```python
from build123d import *

# Parameters (mm, degrees)
BOSS_EXTRUDE1_DEPTH = 59
FILLET1_R           = 1.5
SKETCH2_W           = 8.5
SKETCH2_H           = 4
CUT_EXTRUDE1_DEPTH  = 145.392693721
LPATTERN1_COUNT     = 15
LPATTERN1_PITCH     = 4.8
SKETCH3_W           = 104
SKETCH3_H           = 71.9
BOSS_EXTRUDE2_DEPTH = 22.5
SKETCH4_W           = 35
SKETCH4_H           = 3.5
CUT_EXTRUDE2_DEPTH  = 1
CUT_EXTRUDE3_REACH  = 104.011
SKETCH8_W           = 11.8
SKETCH8_H           = 90
CUT_EXTRUDE4_DEPTH  = 1
SKETCH9_W           = 9
SKETCH9_H           = 30.5
SKETCH9_H_2         = 31.5
BOSS_EXTRUDE4_DEPTH = 2.8
SKETCH10_W          = 9.9
SKETCH10_H          = 21
BOSS_EXTRUDE5_DEPTH = 1
SKETCH11_R          = 1.5
BOSS_EXTRUDE6_DEPTH = 1
FILLET2_R           = 1


# Read off the part's stored shape, not the designer's step: Dome1, Dome2
with BuildPart() as part:
    # Sketch1 → Boss-Extrude1 (new, symmetric)
    with BuildSketch(Plane.XY):
        Polygon((0, 0), (35, 0), (35, 75.5), (23.5, 75.5), (23.5, 3.5), (0, 3.5), align=None)
    extrude(amount=BOSS_EXTRUDE1_DEPTH, both=True)

    # Fillet1
    fillet1_edges = [part.edges().sort_by_distance(p)[0] for p in [
        (35, 37.75, 59),
        (0, 1.75, 59),
        (35, 37.75, -59),
        (0, 1.75, -59),
    ]]
    fillet(fillet1_edges, radius=FILLET1_R)

    # Sketch2 → Cut-Extrude1 (cut, through all)
    with BuildSketch(Plane.XY.offset(59)):
        with Locations((30.75, 5.5)):
            Rectangle(SKETCH2_W, SKETCH2_H)
    cut_extrude1 = extrude(amount=-CUT_EXTRUDE1_DEPTH, mode=Mode.SUBTRACT)

    # LPattern1: Cut-Extrude1 ×15
    with Locations(*[(0, i * LPATTERN1_PITCH, 0) for i in range(1, LPATTERN1_COUNT)]):
        add(cut_extrude1, mode=Mode.SUBTRACT)

    # Sketch3 → Boss-Extrude2 (add)
    with BuildSketch(Plane.ZY.offset(-23.5)):
        with Locations((0, 39.45)):
            Rectangle(SKETCH3_W, SKETCH3_H)
    extrude(amount=BOSS_EXTRUDE2_DEPTH)

    # Sketch4 → Cut-Extrude2 (cut)
    with BuildSketch(Plane.ZY):
        with Locations((0, 1.75)):
            Rectangle(SKETCH4_W, SKETCH4_H)
    extrude(amount=-CUT_EXTRUDE2_DEPTH, mode=Mode.SUBTRACT)

    # Sketch5 → Cut-Extrude3 (cut, up to next)
    with BuildSketch(Plane.XZ, mode=Mode.PRIVATE) as cut_extrude3_sk1:
        with BuildLine():
            Line((12.75, 59), (12.75, 56))
            ThreePointArc((12.75, 56), (10.5, 53.75), (8.25, 56))
            Line((8.25, 56), (8.25, 59))
            ThreePointArc((8.25, 59), (10.5, 61.25), (12.75, 59))
        make_face()
    cut_extrude3_tool1 = extrude(cut_extrude3_sk1.sketch, amount=-CUT_EXTRUDE3_REACH, mode=Mode.PRIVATE) & part.part
    # Sketch5 → Cut-Extrude3 (cut, up to next)
    with BuildSketch(Plane.XZ, mode=Mode.PRIVATE) as cut_extrude3_sk2:
        with BuildLine():
            Line((12.75, -59), (12.75, -56))
            ThreePointArc((12.75, -56), (10.5, -53.75), (8.25, -56))
            Line((8.25, -56), (8.25, -59))
            ThreePointArc((8.25, -59), (10.5, -61.25), (12.75, -59))
        make_face()
    cut_extrude3_tool2 = extrude(cut_extrude3_sk2.sketch, amount=-CUT_EXTRUDE3_REACH, mode=Mode.PRIVATE) & part.part
    add(cut_extrude3_tool1.solids().sort_by_distance((10.5, 0, 57.5))[0], mode=Mode.SUBTRACT)
    add(cut_extrude3_tool2.solids().sort_by_distance((10.5, 0, -57.5))[0], mode=Mode.SUBTRACT)

    # Sketch8 → Cut-Extrude4 (cut)
    with BuildSketch(Plane(origin=(0, 75.4, 0), x_dir=(1, 0, 0), z_dir=(0, 1, 0))):
        with Locations((10.2, 0)):
            Rectangle(SKETCH8_W, SKETCH8_H)
    extrude(amount=-CUT_EXTRUDE4_DEPTH, mode=Mode.SUBTRACT)

    # Sketch9 → Boss-Extrude4 (add)
    with BuildSketch(Plane(origin=(0, 74.4, 0), x_dir=(1, 0, 0), z_dir=(0, 1, 0))):
        with Locations((10.2, -28.65)):
            Rectangle(SKETCH9_W, SKETCH9_H)
        with Locations((10.2, 24.25)):
            Rectangle(SKETCH9_W, SKETCH9_H_2)
    extrude(amount=BOSS_EXTRUDE4_DEPTH)

    # Sketch10 → Boss-Extrude5 (add)
    with BuildSketch(Plane(origin=(0, 74.4, 0), x_dir=(1, 0, 0), z_dir=(0, 1, 0))):
        with Locations((10.25, -2.4)):
            Rectangle(SKETCH10_W, SKETCH10_H)
    extrude(amount=BOSS_EXTRUDE5_DEPTH)

    # Sketch11 → Boss-Extrude6 (add)
    with BuildSketch(Plane(origin=(0, 74.4, 0), x_dir=(1, 0, 0), z_dir=(0, 1, 0))):
        with Locations(Location((6.8, 42.5, 0), (0, 0, 270))):
            Circle(SKETCH11_R)
        with Locations(Location((10.8, 42.5, 0), (0, 0, 270))):
            Circle(SKETCH11_R)
    extrude(amount=BOSS_EXTRUDE6_DEPTH)

    # Dome1 outline → Dome1 (revolve)
    with BuildSketch(Plane(origin=(10.8, 0, -42.5), x_dir=(1, 0, 0), z_dir=(0, 0, 1))):
        with BuildLine():
            Line((0, 75.4), (1.5, 75.399999999))
            ThreePointArc((1.5, 75.399999999), (1.060660172, 76.460660171), (0, 76.9))
            Line((0, 76.9), (0, 75.4))
        make_face()
    revolve(axis=Axis((10.8, 0, -42.5), (0, 1, 0)))

    # Dome2 outline → Dome2 (revolve)
    with BuildSketch(Plane(origin=(6.8, 0, -42.5), x_dir=(1, 0, 0), z_dir=(0, 0, 1))):
        with BuildLine():
            Line((0, 75.4), (1.5, 75.399999999))
            ThreePointArc((1.5, 75.399999999), (1.060660172, 76.460660171), (0, 76.9))
            Line((0, 76.9), (0, 75.4))
        make_face()
    revolve(axis=Axis((6.8, 0, -42.5), (0, 1, 0)))

    # Fillet2
    fillet2_edges = [part.edges().sort_by_distance(p)[0] for p in [
        (1, 75.4, 0),
        (12.25, 75.4, 52),
        (1, 39.45, 52),
        (1, 39.45, -52),
        (12.25, 75.4, -52),
    ]]
    fillet(fillet2_edges, radius=FILLET2_R)


solid = part.part
```
CAD build for the part. Positions are in the model's coordinates, mm. A direction names the side the tool comes from. Give positions to 0.01 mm unless a question says otherwise; leave off trailing zeros. Order: outer loops, then holes, each group sorted by start corner. A loop starts at its lowest first (then second) coordinate and runs counter-clockwise, first axis right, second up. Notation, with made-up numbers: M -19.75,-4 L 4.25,-4 A24 cw 4.25,30 Z; hole C -16.75,74.25 d6. An arc over 180 degrees is marked long. Put each result on its own line as item: value. Start each with the question number.
(1) Drill centre lines: line 1 along X through (y, z) = (66, 2.5); line 2 along Z through (x, y) = (10, 28.5); line 3 along Y through (x, z) = (5, 48.5). Where is each one in solid material? Low to high.
(2) Flat gauge pins, fed straight in: pin 1 Ø9.5 at (x, z) = (29, 20.5) entering from -Y; pin 2 Ø2 at (y, z) = (73.5, 6.5) entering from +X; pin 3 Ø1.5 at (y, z) = (59, 41.5) entering from -X; pin 4 Ø1.1 at (x, y) = (12.5, 75) entering from +Z. Where does each tip first touch, or does it go through?
(3) Which spindle directions (+Z, -Z, +X, -X, +Y, -Y) get a long thin tool onto all of the face, cutting with end or side? Do faces 4 (the flat face through (31, 12.3, 1)), 5 (the flat face through (10.1, 3.5, -53.5)), 6 (the flat face through (14.7, 76, 29)). Say none if no direction does.
(4) Mould opens along Y. For faces 1 (the flat face through (17, 0, 1)), 2 (the flat face through (35, 2, 1)), 3 (the flat face through (26.5, 10, 1)) say: +Y half, -Y half, draft (parallel to the pull), parting line (faces both ways), or undercut.
(5) Saw through at A-A, the plane y = 63.5. Write the cut outline in (x, z), then the cut area to 3 significant figures.
Check result:
1. line 1: x = 1 to 26.5
1. line 2: z = -52 to 52
1. line 3: y = 0 to 75.4
2. pin 1: stops at y = 0
2. pin 2: stops at x = 26.5
2. pin 3: stops at x = 1
2. pin 4: stops at z = 52
3. face 4: +Z, -Z, +X
3. face 5: -Z, -X, +Y
3. face 6: +Y
4. face 1: -Y half
4. face 2: draft
4. face 3: undercut
5. outline: M 1,-51 A1 ccw 2,-52 L 23.5,-52 L 23.5,-59 L 26.5,-59 L 26.5,59 L 23.5,59 L 23.5,52 L 2,52 A1 ccw 1,51 Z
5. area: 2,690 mm2
